Check sheet for the modelled part. Datum: model origin and axes. Units: mm. Face numbers are marked on the shaded views. A direction names the side the tool comes from. Round coordinates to 2 decimals unless told otherwise and drop trailing zeros. Order: outer loops, then holes, each group sorted by start corner. A loop starts at its lowest first (then second) coordinate and runs counter-clockwise, first axis right, second up. Notation, with made-up numbers: (81.25, 23.5) -> (121.25, 23.5) arc R23 ccw to (121.25, 58.5) -> close; hole circle Ø7 at (-28, -31). An arc over 180 degrees is marked (long way). Use CSV: the item, a comma, the result in double quotes.
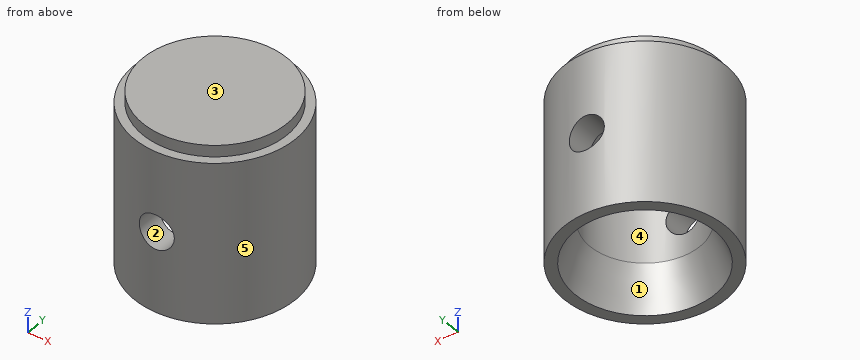
Solid Edge part; units mm, degrees
sketch "Sketch1" plane through (0, 0, 0) normal (0, -1, 0) x (1, 0, 0)
  line L0 (-4.75, 38.4552) -> (-4.75, 31.0416)
  line L1 (-4.75, 31.0416) -> (-6.0553, 27.4552)
  line L2 (-7, 27.4552) -> (-6.0553, 27.4552)
  line L3 (-7, 41.4552) -> (-7, 27.4552)
  line L4 (-6.25, 41.4552) -> (-7, 41.4552)
  line L5 (-6.25, 42.4552) -> (-6.25, 41.4552)
  line L6 (0, 42.4552) -> (-6.25, 42.4552)
  line L7 (0, 42.4552) -> (0, 41.3093)
  line L8 (0, 41.3093) -> (-4.75, 38.4552)
revolve "RevolvedProtrusion1" add sketch "Sketch1" angle 360 about axis through (0, 0, 42.4552) along (0, 0, -1)
hole "Hole1" at (0, 0, 34.4552) direction (0, -1, 0) diameter 3 end through all both ways yes
Q1. Scan lines: L1, parallel to X at y = 2.75, z = 30; L2, parallel to X at y = -4.75, z = 33.25; L3, parallel to Y at x = -0.25, z = 31. Record each from-to range of solid material in increasing order.
Result sheet:
L1,"x = -6.44 to -4.33, 4.33 to 6.44"
L2,"x = -5.14 to -0.89, 0.89 to 5.14"
L3,"y = -7 to -4.76, 4.76 to 7"
Q2. Sectioned sample at C-C, the plane x = 0.75. State how many separate pieces and enclosed holes the cut face has, then the cut area to 3 significant figures.
Result sheet:
separate pieces,"3"
enclosed holes,"0"
area,"75.0 mm^2"
Q3. Access from +Z, -Z, +X, -X, +Y, -Y to the whole of each face (thin tool, end or side, straight path). Record for the marked faces 4 and 5.
Result sheet:
face 4,"-Z"
face 5,"+Z, -Z"
Q4. Sectioned sample at B-B, the plane z = 32. Enter the section's corners in (x, y).
Result sheet:
outline,"circle Ø14 at (0, 0); hole circle Ø9.5 at (0, 0)"
Q5. Sectioned sample at A-A, the plane z = 35. Enter the section's corners in (x, y), then the cut area to 3 significant figures.
Result sheet:
outline,"(-1.4, -6.86) -> (-1.4, -4.54) arc R4.75 cw to (-1.4, 4.54) -> (-1.4, 6.86) arc R7 ccw to start; (1.4, -6.86) arc R7 ccw to (1.4, 6.86) -> (1.4, 4.54) arc R4.75 cw to (1.4, -4.54) -> close"
area,"70.4 mm^2"
Q6. Go/stop test with flat-tipped pins: pin 1 (1.5 mm diameter, centred on y = -4, z = 36, fed in from +X); pin 2 (5 mm diameter, centred on x = -4.5, z = 34, fed in from +Y); pin 3 (1 mm diameter, centred on y = 1, z = 32.5, fed in from +X). Record where each tip stops, or that it passes through.
Result sheet:
pin 1,"stops at x = 6.2"
pin 2,"stops at y = 6.71"
pin 3,"stops at x = 6.98"
Q7. Mould release check, pull along Z, two halves, no side actions. Record for the marked faces 1, 2 and 3: pulls with the +Z half, pulls with the -Z half, needs draft (parallel to the pull), parting line crosses it, or undercut.
Result sheet:
face 1,"pulls with the -Z half"
face 2,"undercut"
face 3,"pulls with the +Z half"
